Geometry check sheet. Reference: the model listing, model coordinates, mm. A direction names the side the tool comes from. Round coordinates to 2 decimals unless told otherwise and drop trailing zeros. Loops run counter-clockwise (first coordinate to the right, second up) from the corner with the lowest first, then second, coordinate; pieces in that order, holes last. Notation, with made-up numbers: (4, 59) -> (44, 59) arc R23 ccw to (44, 93) -> close; hole circle Ø10 at (-12, 88). An arc over 180 degrees is marked (long way). Use one line per item in the form item = value.
from build123d import *

# Parameters (mm, degrees)
SKETCH1_R           = 11
BOSS_EXTRUDE1_DEPTH = 3.5
SKETCH2_R           = 3.5
CUT_EXTRUDE2_DEPTH  = 8
SKETCH3_R           = 8.75
SKETCH3_R_2         = 6
CUT_EXTRUDE4_DEPTH  = 1.8
FILLET1_R           = 0.5


with BuildPart() as part:
    # Sketch1 → Boss-Extrude1 (new body, symmetric)
    with BuildSketch(Plane(origin=(0, 0, 0), x_dir=(1, 0, 0), z_dir=(0, 1, 0))):
        Circle(SKETCH1_R)
    extrude(amount=BOSS_EXTRUDE1_DEPTH, both=True)

    # Sketch2 → Cut-Extrude2 (cut, through all)
    with BuildSketch(Plane(origin=(0, 3.5, 0), x_dir=(1, 0, 0), z_dir=(0, 1, 0))):
        Circle(SKETCH2_R)
    extrude(amount=-CUT_EXTRUDE2_DEPTH, mode=Mode.SUBTRACT)

    # Sketch3 → Cut-Extrude4 (cut)
    with BuildSketch(Plane(origin=(0, 3.5, 0), x_dir=(1, 0, 0), z_dir=(0, 1, 0))):
        Circle(SKETCH3_R)
        Circle(SKETCH3_R_2, mode=Mode.SUBTRACT)
    cut_extrude4 = extrude(amount=-CUT_EXTRUDE4_DEPTH, mode=Mode.SUBTRACT)

    # Mirror1: Cut-Extrude4 across plane
    add(cut_extrude4.mirror(Plane.ZX), mode=Mode.SUBTRACT)

    # Fillet1
    fillet1_edges = [part.edges().sort_by_distance(p)[0] for p in [
        (-8.75, 3.5, 0),
        (-11, -3.5, 0),
        (-8.75, -3.5, 0),
        (-11, 3.5, 0),
    ]]
    fillet(fillet1_edges, radius=FILLET1_R)


solid = part.part
1. Section check D-D (y = -0.25). Record the boundary of the cut face in (x, z), then the cut area to 3 significant figures.
Return value:
outline = circle Ø22 at (0, 0); hole circle Ø7 at (0, 0)
area = 342 mm2
2. Material ranges on line 1 along X through (y, z) = (-2.45, 0); line 2 along X through (y, z) = (-1, 0), recorded low to high.
Return value:
line_1 = -11 to -8.75, -6 to -3.5, 3.5 to 6, 8.75 to 11
line_2 = -11 to -3.5, 3.5 to 11
3. Gauge pin test, flat ends, axial feed: pin 1 (3 mm diameter, centred on x = -3.5, y = 1, fed in from -Z); pin 2 (2 mm diameter, centred on x = 8, y = 0, fed in from -Z); pin 3 (3 mm diameter, centred on x = 2.5, y = -1.5, fed in from +Z). Record the tip position at first contact, or that the pin passes through.
Return value:
pin_1 = -10.82
pin_2 = -8.49
pin_3 = 10.95
4. Mould release check, pull along Z, two halves, no side actions. Record for faces 4 (the flat face through (-2, 1.7, 6)), 5 (the flat face through (3, 3.5, 3)), 6 (the cylindrical face through (-2.38, 0.04, 10.74)): released by +Z, released by -Z, zero draft, split by the parting line, or undercut.
Return value:
face_4 = undercut
face_5 = zero draft
face_6 = split by the parting line
5. Section check C-C (y = 2.5). Record the boundary of the cut face in (x, z), then the cut area to 3 significant figures.
Return value:
outline = circle Ø22 at (0, 0); circle Ø12 at (0, 0); hole circle Ø17.5 at (0, 0); hole circle Ø7 at (0, 0)
area = 214 mm2
6. Tool access check on faces 1 (the flat face through (3, -3.5, 3)), 2 (the cylindrical face through (-6, -3, 0)), 3 (the cylindrical face through (-6.944, 2.359, 5.324)). Record the directions out of +Z, -Z, +X, -X, +Y, -Y that give a thin tool (end or side, any length) a straight path to the whole face; none if there is none.
Return value:
face_1 = +Z, -Z, +X, -X, -Y
face_2 = -Y
face_3 = +Y
